```python
from build123d import *

# Parameters (mm, degrees)
F0_R     = 10
F0_R_2   = 0.625
F1_DEPTH = 2


with BuildPart() as f1:
    # F0 (on Top) → F1 (new body)
    with BuildSketch(Plane.XY):
        Circle(F0_R)
        with BuildLine():
            Line((-0.625, -2.52178), (-0.625, -7.833223))
            ThreePointArc((-0.625, -7.833223), (-0.993781, -8.608827), (-1.828125, -8.812375))
            ThreePointArc((-1.828125, -8.812375), (-6.363961, -6.363961), (-8.812375, -1.828125))
            ThreePointArc((-8.812375, -1.828125), (-8.608827, -0.993781), (-7.833223, -0.625))
            Line((-7.833223, -0.625), (-2.52178, -0.625))
            ThreePointArc((-2.52178, -0.625), (-2.043067, -0.747029), (-1.681187, -1.083333))
            ThreePointArc((-1.681187, -1.083333), (-1.414214, -1.414214), (-1.083333, -1.681187))
            ThreePointArc((-1.083333, -1.681187), (-0.747029, -2.043067), (-0.625, -2.52178))
        make_face(mode=Mode.SUBTRACT)
        with BuildLine():
            Line((2.52178, -0.625), (7.833223, -0.625))
            ThreePointArc((7.833223, -0.625), (8.608827, -0.993781), (8.812375, -1.828125))
            ThreePointArc((8.812375, -1.828125), (6.363961, -6.363961), (1.828125, -8.812375))
            ThreePointArc((1.828125, -8.812375), (0.993781, -8.608827), (0.625, -7.833223))
            Line((0.625, -7.833223), (0.625, -2.52178))
            ThreePointArc((0.625, -2.52178), (0.747029, -2.043067), (1.083333, -1.681187))
            ThreePointArc((1.083333, -1.681187), (1.414214, -1.414214), (1.681187, -1.083333))
            ThreePointArc((1.681187, -1.083333), (2.043067, -0.747029), (2.52178, -0.625))
        make_face(mode=Mode.SUBTRACT)
        with BuildLine():
            ThreePointArc((-0.625, 2.52178), (-0.747029, 2.043067), (-1.083333, 1.681187))
            ThreePointArc((-1.083333, 1.681187), (-1.414214, 1.414214), (-1.681187, 1.083333))
            ThreePointArc((-1.681187, 1.083333), (-2.043067, 0.747029), (-2.52178, 0.625))
            Line((-2.52178, 0.625), (-7.833223, 0.625))
            ThreePointArc((-7.833223, 0.625), (-8.608827, 0.993781), (-8.812375, 1.828125))
            ThreePointArc((-8.812375, 1.828125), (-6.363961, 6.363961), (-1.828125, 8.812375))
            ThreePointArc((-1.828125, 8.812375), (-0.993781, 8.608827), (-0.625, 7.833223))
            Line((-0.625, 7.833223), (-0.625, 2.52178))
        make_face(mode=Mode.SUBTRACT)
        Circle(F0_R_2, mode=Mode.SUBTRACT)
        with BuildLine():
            ThreePointArc((1.828125, 8.812375), (6.363961, 6.363961), (8.812375, 1.828125))
            ThreePointArc((8.812375, 1.828125), (8.608827, 0.993781), (7.833223, 0.625))
            Line((7.833223, 0.625), (2.52178, 0.625))
            ThreePointArc((2.52178, 0.625), (2.043067, 0.747029), (1.681187, 1.083333))
            ThreePointArc((1.681187, 1.083333), (1.414214, 1.414214), (1.083333, 1.681187))
            ThreePointArc((1.083333, 1.681187), (0.747029, 2.043067), (0.625, 2.52178))
            Line((0.625, 2.52178), (0.625, 7.833223))
            ThreePointArc((0.625, 7.833223), (0.993781, 8.608827), (1.828125, 8.812375))
        make_face(mode=Mode.SUBTRACT)
    extrude(amount=F1_DEPTH)


solid = f1.part
```
Work out the finished part from the listing and answer in its coordinate system (mm). Give positions to 0.01 mm unless a question says otherwise; leave off trailing zeros. Order: outer loops, then holes, each group sorted by start corner. A loop starts at its lowest first (then second) coordinate and runs counter-clockwise, first axis right, second up. Notation, with made-up numbers: (43.25, 86) -> (101.25, 86) arc R20 cw to (101.25, 104) -> close; hole circle Ø8 at (50, 34). An arc over 180 degrees is marked (long way). Answer as CSV lines item,"result". Start each with the question number.
(1) Each of these flat-tipped pins is pushed along its axis until it touches: pin 1 Ø0.6 at (x, z) = (-4.5, 1.5) entering from +Y; pin 2 Ø1 at (y, z) = (-4.5, 1) entering from +X; pin 3 Ø0.6 at (y, z) = (-5.5, 1) entering from -X. Where does it stop, or does it pass through?
(2) Section A-A, the plane z = 0.25 is taken. Give the number of separate pieces and of enclosed holes in the cut face, plus the area to 3 significant figures.
(3) Section D-D, the plane x = 6.75 is taken. Write down the section's boundary in (y, z) (3 decimals), plus the area to 3 significant figures.
(4) Section B-B, the plane x = 0 is taken. Write down the section's boundary in (y, z) (3 decimals).
(5) For a pull along Y with two mould halves and no side action, classify faces 1 (the flat face through (0, -2, 0)), 2 (the cylindrical face through (-6.31, -6.42, 0.99)), 3 (the flat face through (-0.625, -5, 1)) as released by +Y, released by -Y, zero draft, split by the parting line, or undercut.
(6) Consider line 1 along Y through (x, z) = (0, 0.45) (3 decimals); line 2 along X through (y, z) = (-1.75, 0.35); line 3 along X through (y, z) = (1.5, 0.8). Determine where each line is inside the solid, lowest interval first.
Entries:
1,pin 1,"y = 9.08"
1,pin 2,"x = 9.17"
1,pin 3,"x = -8.54"
2,separate pieces,"1"
2,enclosed holes,"5"
2,area,"109 mm²"
3,outline,"(-7.378, 0) -> (-5.953, 0) -> (-5.953, 2) -> (-7.378, 2) -> close; (-0.625, 0) -> (0.625, 0) -> (0.625, 2) -> (-0.625, 2) -> close; (5.953, 0) -> (7.378, 0) -> (7.378, 2) -> (5.953, 2) -> close"
3,area,"8.20 mm²"
4,outline,"(-10, 0) -> (-0.625, 0) -> (-0.625, 2) -> (-10, 2) -> close; (0.625, 0) -> (10, 0) -> (10, 2) -> (0.625, 2) -> close"
5,face 1,"zero draft"
5,face 2,"undercut"
5,face 3,"undercut"
6,line 1,"-10 to -0.625, 0.625 to 10"
6,line 2,"-9.85 to -8.83, -0.99 to 0.99, 8.83 to 9.85"
6,line 3,"-9.89 to -8.83, -1.32 to 1.32, 8.83 to 9.89"
